Geometry: final body of the model. Coordinates: model frame, mm. A direction names the side the tool comes from. Round coordinates to 2 decimals unless told otherwise and drop trailing zeros. Loops run counter-clockwise (first coordinate to the right, second up) from the corner with the lowest first, then second, coordinate; pieces in that order, holes last. Notation, with made-up numbers: M -20,17.5 L 7,17.5 A15 ccw 7,31.5 Z; hole C 60,-33.75 d11. An arc over 180 degrees is marked long. Return JSON: item names as keys, results as strings.
from build123d import *

# Parameters (mm, degrees)
F0_W     = 90
F0_H     = 90
F0_R     = 1.8
F0_R_2   = 2.15
F1_DEPTH = 1.5
F2_SIZE2 = 1
F2_SIZE  = 1
F3_SIZE  = 0.5


with BuildPart() as f1:
    # F0 (on Top) → F1 (new body)
    with BuildSketch(Plane.XY):
        Rectangle(F0_W, F0_H)
        with Locations((-37.2, -37.2)):
            Circle(F0_R, mode=Mode.SUBTRACT)
        with Locations((-24.85, -24.85)):
            Circle(F0_R_2, mode=Mode.SUBTRACT)
        with Locations((37.2, -37.2)):
            Circle(F0_R, mode=Mode.SUBTRACT)
        with Locations((24.85, -24.85)):
            Circle(F0_R_2, mode=Mode.SUBTRACT)
        with Locations((-24.85, 24.85)):
            Circle(F0_R_2, mode=Mode.SUBTRACT)
        with Locations((-37.2, 37.2)):
            Circle(F0_R, mode=Mode.SUBTRACT)
        with BuildLine():
            Line((-5.408327, 29), (5.408327, 29))
            ThreePointArc((5.408327, 29), (20.85965, 20.85965), (29, 5.408327))
            Line((29, 5.408327), (29, -5.408327))
            ThreePointArc((29, -5.408327), (20.85965, -20.85965), (5.408327, -29))
            Line((5.408327, -29), (-5.408327, -29))
            ThreePointArc((-5.408327, -29), (-20.85965, -20.85965), (-29, -5.408327))
            Line((-29, -5.408327), (-29, 5.408327))
            ThreePointArc((-29, 5.408327), (-20.85965, 20.85965), (-5.408327, 29))
        make_face(mode=Mode.SUBTRACT)
        with Locations((24.85, 24.85)):
            Circle(F0_R_2, mode=Mode.SUBTRACT)
        with Locations((37.2, 37.2)):
            Circle(F0_R, mode=Mode.SUBTRACT)
    extrude(amount=F1_DEPTH)

    # F2
    f2_edges = [f1.edges().sort_by_distance(p)[0] for p in [
        (-39, 37.2, 1.5),
        (35.4, 37.2, 1.5),
        (35.4, -37.2, 1.5),
        (-39, -37.2, 1.5),
    ]]
    chamfer(f2_edges, length=F2_SIZE, length2=F2_SIZE2)

    # F3
    f3_edges = [f1.edges().sort_by_distance(p)[0] for p in [
        (0, -45, 0),
        (-45, 0, 0),
        (45, 0, 0),
        (0, 45, 0),
        (-45, 0, 1.5),
        (0, -45, 1.5),
        (45, 0, 1.5),
        (0, 45, 1.5),
        (-20.85965, -20.85965, 0),
        (-20.85965, -20.85965, 1.5),
        (0, -29, 0),
        (0, -29, 1.5),
        (20.85965, -20.85965, 0),
        (20.85965, -20.85965, 1.5),
        (-29, 0, 0),
        (-29, 0, 1.5),
        (-20.85965, 20.85965, 1.5),
        (-20.85965, 20.85965, 0),
        (20.85965, 20.85965, 1.5),
        (29, 0, 1.5),
        (0, 29, 1.5),
        (29, 0, 0),
        (20.85965, 20.85965, 0),
        (0, 29, 0),
    ]]
    chamfer(f3_edges, length=F3_SIZE)


solid = f1.part
Q1. Reachability of faces 1 (the conical face through (-21.131, 20.778, 1.135)), 2 (the cylindrical face through (20.683, 21.034, 0.746)), 3 (the conical face through (20.778, 21.131, 0.365)) from +Z, -Z, +X, -X, +Y, -Y: full face, straight path, thin tool, end or side. Return the list, or none.
Determined:
{"face 1": "+Z", "face 2": "+Z, -Z", "face 3": "-Z"}
Q2. Section query A-A (x = -37.2). Output: boundary loops of the cut face in (y, z).
Determined:
{"outline": "M -45,0.5 L -44.5,0 L -39,0 L -39,0.5 L -40,1.5 L -44.5,1.5 L -45,1 Z; M -35.4,0 L 35.4,0 L 35.4,0.5 L 34.4,1.5 L -34.4,1.5 L -35.4,0.5 Z; M 39,0 L 44.5,0 L 45,0.5 L 45,1 L 44.5,1.5 L 40,1.5 L 39,0.5 Z"}
Q3. Material intervals for L1, parallel to Y at x = 37.2, z = 0.4; L2, parallel to X at y = 25, z = 1.05; L3, parallel to Y at x = -24.5, z = 1.1, sorted ascending.
Determined:
{"L1": "y = -44.9 to -39, -35.4 to 35.4, 39 to 44.9", "L2": "x = -44.95 to -26.99, -22.71 to -15.75, 15.75 to 22.71, 26.99 to 44.95", "L3": "y = -44.9 to -26.97, -22.73 to -16.61, 16.61 to 22.73, 26.97 to 44.9"}
Q4. Section query C-C (y = -24.85). State how many separate pieces and enclosed holes the cut face has, plus the area to 3 significant figures.
Determined:
{"separate pieces": "4", "enclosed holes": "0", "area": "73.0 mm^2"}
Q5. Pin query (flat end, axial travel): pin 1 (4 mm diameter, centred on x = 37.2, y = -37.2, fed in from +Z). Return the tip coordinate at first contact, or that it passes through.
Determined:
{"pin 1": "stops at z = 0.7"}
Q6. Pull-direction query (Y, two-part tool) for faces 4 (the conical face through (20.778, 21.131, 1.135)), 5 (the cylindrical face through (-25.13, 26.98, 0.74)), 6 (the flat face through (-1, 30, 0)); classes: pulls with the +Y half, pulls with the -Y half, needs draft (parallel to the pull), parting line crosses it, or undercut.
Determined:
{"face 4": "undercut", "face 5": "undercut", "face 6": "needs draft"}
